Work out the finished part from the listing and answer in its coordinate system (mm). A direction names the side the tool comes from. Coordinates: 2 decimals unless noted, no trailing zeros. Order: outer loops, then holes, each group sorted by start corner. A loop starts at its lowest first (then second) coordinate and runs counter-clockwise, first axis right, second up. Notation, with made-up numbers: (1.5, -15.75) -> (27.5, -15.75) arc R14 cw to (27.5, 5.25) -> close; hole circle Ø6 at (73, 28.5). An arc over 180 degrees is marked (long way). Use one line per item in the form item = value.
from build123d import *

# Parameters (mm, degrees)
F0_W     = 15
F0_H     = 12
F1_DEPTH = 2
F2_W     = 2
F2_H     = 4
F3_DEPTH = 3.05
F4_R     = 0.4
F5_DEPTH = 25
F6_R     = 0.99999
F7_R     = 1
F8_DEPTH = 25


# Not quite as in the source:
# - a fillet or chamfer is up to 0.001 mm smaller than in the source, because OpenCascade refuses the exact size


with BuildPart() as f1:
    # F0 (on Front) → F1 (new body)
    with BuildSketch(Plane.XZ):
        Rectangle(F0_W, F0_H)
    extrude(amount=F1_DEPTH)

    # F2 (on face) → F3 (join)
    with BuildSketch(Plane.XZ.offset(2)):
        with Locations((6.5, 4)):
            Rectangle(F2_W, F2_H)
        with Locations((6.5, -4)):
            Rectangle(F2_W, F2_H)
    extrude(amount=F3_DEPTH)

    # F4 (on face) → F5 (cut)
    with BuildSketch(Plane(origin=(0, 0, -6), x_dir=(1, 0, 0), z_dir=(0, 0, -1))):
        with Locations((6.5, 3.525)):
            Circle(F4_R)
    extrude(amount=-F5_DEPTH, mode=Mode.SUBTRACT)

    # F6 (radius 1 in the source; OpenCascade refuses exactly that, so slightly less here)
    f6_edges = [f1.edges().sort_by_distance(p)[0] for p in [
        (7.5, -5.05, 4),
        (5.5, -5.05, 4),
        (7.5, -5.05, -4),
        (5.5, -5.05, -4),
    ]]
    fillet(f6_edges, radius=F6_R)

    # F7 (on face) → F8 (cut)
    with BuildSketch(Plane(origin=(0, 0, 0), x_dir=(-1, 0, 0), z_dir=(0, 1, 0))):
        with Locations((0, 3.5)):
            Circle(F7_R)
        with Locations((0, -3.5)):
            Circle(F7_R)
    extrude(amount=-F8_DEPTH, mode=Mode.SUBTRACT)


solid = f1.part
(1) Section C-C on z = -3.5 is taken. Count the separate pieces of the cut face and the enclosed holes in it, plus the area to 3 significant figures.
Data:
separate_pieces = 2
enclosed_holes = 1
area = 31.2 mm²
(2) Which of the six approach directions +Z, -Z, +X, -X, +Y, -Y give full straight-line access (tool end or side, diameter ignored) to faces 1 (the cylindrical face through (-0.954, -0.986, -3.2)), 2 (the flat face through (7, -3, -2)), 3 (the flat face through (5.5, -3, 4))?
Data:
face_1 = +Y, -Y
face_2 = +X, -X, -Y
face_3 = +Z, -Z, -X, -Y
(3) Section B-B on x = 0 is taken. Write down the section's boundary in (y, z), plus the area to 3 significant figures.
Data:
outline = (-2, -6) -> (0, -6) -> (0, -4.5) -> (-2, -4.5) -> close; (-2, -2.5) -> (0, -2.5) -> (0, 2.5) -> (-2, 2.5) -> close; (-2, 4.5) -> (0, 4.5) -> (0, 6) -> (-2, 6) -> close
area = 16.0 mm²
(4) The mould has two halves that part along Z. Classify faces 4 (the flat face through (5.5, -3, -4)), 5 (the flat face through (7, -3, 2)), 6 (the flat face through (0, -1, 6)), 7 (the flat face through (0, -1, -6)): released by +Z, released by -Z, zero draft, split by the parting line, or undercut.
Data:
face_4 = zero draft
face_5 = undercut
face_6 = released by +Z
face_7 = released by -Z
(5) Straight lines are drawn through the part: line 1 along Z through (x, y) = (0, -1.45); line 2 along Y through (x, z) = (-6.75, 2.75); line 3 along X through (y, z) = (-3, -4.5). For each, find the intervals that lie inside material, in ascending order.
Data:
line_1 = -6 to -4.5, -2.5 to 2.5, 4.5 to 6
line_2 = -2 to 0
line_3 = 5.5 to 7.5
(6) Each of these flat-tipped pins is pushed along its axis until it touches: P1, Ø2, axis at x = -5, z = 1, coming from the -Y side; P2, Ø5, axis at x = 3.5, z = 4, coming from the -Y side; P3, Ø5, axis at x = 3.5, z = 1, coming from the -Y side. Where does it stop, or does it pass through?
Data:
P1 = -2
P2 = -4.92
P3 = -4.76
(7) Section D-D on y = -0.45 is taken. Write down the section's boundary in (x, z), plus the area to 3 significant figures.
Data:
outline = (-7.5, -6) -> (7.5, -6) -> (7.5, 6) -> (-7.5, 6) -> close; hole circle Ø2 at (0, -3.5); hole circle Ø2 at (0, 3.5)
area = 174 mm²
(8) Section A-A on y = -4.65 is taken. Write down the section's boundary in (x, z).
Data:
outline = (5.7, -6) -> (7.3, -6) -> (7.3, -2) -> (5.7, -2) -> close; (5.7, 2) -> (7.3, 2) -> (7.3, 6) -> (5.7, 6) -> close
